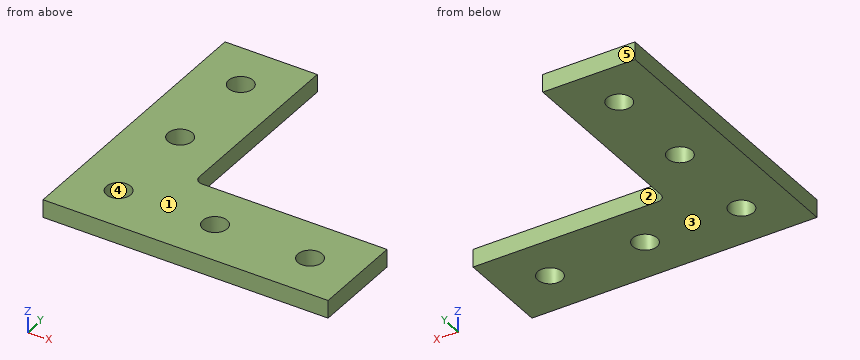
from build123d import *

# Parameters (mm, degrees)
BOSS_EXTRUDE1_DEPTH      = 2.3876
BOSS_EXTRUDE1_DEPTH_BACK = 2.3876
SKETCH4_R                = 3.2639
CUT_EXTRUDE1_DEPTH       = 1
CUT_EXTRUDE1_DEPTH_BACK  = 5.7752


with BuildPart() as part:
    # Sketch3 → Boss-Extrude1 (new body, two sides)
    with BuildSketch(Plane.XY) as boss_extrude1_sk:
        with BuildLine():
            Line((-13.4366, 38.1), (-38.1, 38.1))
            Line((-38.1, 38.1), (-38.1, -38.1))
            Line((-38.1, -38.1), (38.1, -38.1))
            Line((38.1, -38.1), (38.1, -13.4366))
            Line((38.1, -13.4366), (-11.3538, -13.4366))
            ThreePointArc((-11.3538, -13.4366), (-12.826562004, -12.826562004), (-13.4366, -11.3538))
            Line((-13.4366, -11.3538), (-13.4366, 38.1))
        make_face()
    extrude(amount=BOSS_EXTRUDE1_DEPTH)
    extrude(boss_extrude1_sk.sketch, amount=-BOSS_EXTRUDE1_DEPTH_BACK)

    # Sketch4 → Cut-Extrude1 (cut, two sides)
    with BuildSketch(Plane.XY.offset(2.3876)) as cut_extrude1_sk:
        with Locations((-25.7683, 25.4)):
            Circle(SKETCH4_R)
        with Locations((-25.7683, 0)):
            Circle(SKETCH4_R)
        with Locations((0, -25.7683)):
            Circle(SKETCH4_R)
        with Locations((25.4, -25.7683)):
            Circle(SKETCH4_R)
        with Locations((-25.7683, -25.7683)):
            Circle(SKETCH4_R)
    extrude(amount=CUT_EXTRUDE1_DEPTH, mode=Mode.SUBTRACT)
    extrude(cut_extrude1_sk.sketch, amount=-CUT_EXTRUDE1_DEPTH_BACK, mode=Mode.SUBTRACT)


solid = part.part
Geometry: final body of the model. Coordinates: model frame, mm. Face numbers are marked on the shaded views. A direction names the side the tool comes from. Coordinates: 2 decimals unless noted, no trailing zeros. Order: outer loops, then holes, each group sorted by start corner. A loop starts at its lowest first (then second) coordinate and runs counter-clockwise, first axis right, second up.
1) Set-up query: the marked faces 1 and 2. Return all of +Z, -Z, +X, -X, +Y, -Y with unobstructed straight access to the full face (end or side cutting, diameter ignored); none if empty.
Result sheet:
face 1: +Z, +X, -X, +Y, -Y
face 2: +Z, -Z, +X, +Y
2) First-contact query: P1, Ø5, axis at x = -25.77, y = -25.77, coming from the -Z side; P2, Ø2.5, axis at y = 9, z = -1, coming from the +X side. Flat tips, straight axial feed; report the tip coordinate or a pass-through.
Result sheet:
P1: passes through
P2: stops at x = -13.44
3) Section A-A (y = 0). Return loops of the section in (x, z).
Result sheet:
outline: (-38.1, -2.39) - (-29.03, -2.39) - (-29.03, 2.39) - (-38.1, 2.39) - close; (-22.5, -2.39) - (-13.44, -2.39) - (-13.44, 2.39) - (-22.5, 2.39) - close
4) Draft query along Y for the marked faces 3, 4 and 5. Return one class per face: released by +Y, released by -Y, zero draft, split by the parting line, or undercut.
Result sheet:
face 3: zero draft
face 4: undercut
face 5: released by +Y
5) Section D-D (z = -0.85). Return loops of the section in (x, y).
Result sheet:
outline: (-38.1, -38.1) - (38.1, -38.1) - (38.1, -13.44) - (-11.35, -13.44) arc R2.08 cw to (-13.44, -11.35) - (-13.44, 38.1) - (-38.1, 38.1) - close; hole circle Ø6.53 at (-25.77, -25.77); hole circle Ø6.53 at (-25.77, 0); hole circle Ø6.53 at (-25.77, 25.4); hole circle Ø6.53 at (0, -25.77); hole circle Ø6.53 at (25.4, -25.77)
6) Section C-C (x = -27). Return loops of the section in (y, z), then the cut area to 3 significant figures.
Result sheet:
outline: (-38.1, -2.39) - (-28.79, -2.39) - (-28.79, 2.39) - (-38.1, 2.39) - close; (-22.75, -2.39) - (-3.02, -2.39) - (-3.02, 2.39) - (-22.75, 2.39) - close; (3.02, -2.39) - (22.38, -2.39) - (22.38, 2.39) - (3.02, 2.39) - close; (28.42, -2.39) - (38.1, -2.39) - (38.1, 2.39) - (28.42, 2.39) - close
area: 277 mm2
7) Ray query, probe 1 along X at (y, z) = (-26.5, -0.75); probe 2 along Y at (x, z) = (-23.5, 0.9); probe 3 along Y at (x, z) = (6.5, -1.2). Return the intervals inside material, ascending.
Result sheet:
probe 1: x = -38.1 to -28.95, -22.59 to -3.18, 3.18 to 22.22, 28.58 to 38.1
probe 2: y = -38.1 to -28.12, -23.42 to -2.35, 2.35 to 23.05, 27.75 to 38.1
probe 3: y = -38.1 to -13.44
